The model under review builds one solid part; all positions refer to its coordinate system, in mm. Coordinates: 2 decimals unless noted, no trailing zeros. Loops run counter-clockwise (first coordinate to the right, second up) from the corner with the lowest first, then second, coordinate; pieces in that order, holes last. Notation, with made-up numbers: M 8.25,-21 L 32.25,-21 A18 cw 32.25,5 Z; hole C -6.75,-32.5 d3. An arc over 180 degrees is marked long. One line per item, written item: value.
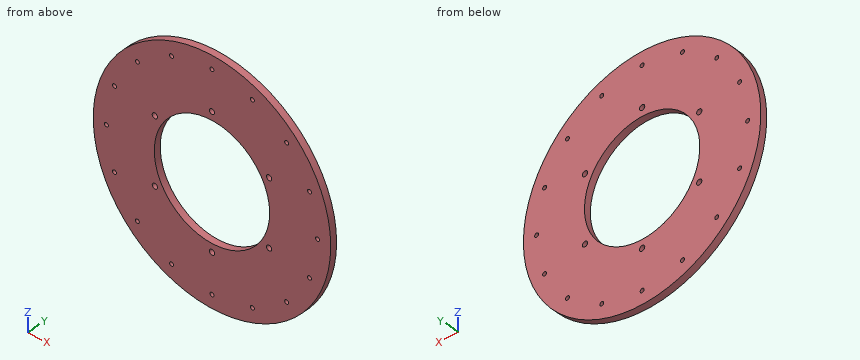
```python
from build123d import *

# Parameters (mm, degrees)
SKETCH1_R           = 180
SKETCH1_R_2         = 87.5
SKETCH1_R_3         = 3
SKETCH1_R_4         = 4
BOSS_EXTRUDE1_DEPTH = 10


with BuildPart() as part:
    # Sketch1 → Boss-Extrude1 (new body)
    with BuildSketch(Plane(origin=(0, 0, 0), x_dir=(1, 0, 0), z_dir=(0, 1, 0))):
        Circle(SKETCH1_R)
        Circle(SKETCH1_R_2, mode=Mode.SUBTRACT)
        with Locations((0, 160)):
            Circle(SKETCH1_R_3, mode=Mode.SUBTRACT)
        with Locations((61.229349178, 147.820725202)):
            Circle(SKETCH1_R_3, mode=Mode.SUBTRACT)
        with Locations((113.13708499, 113.13708499)):
            Circle(SKETCH1_R_3, mode=Mode.SUBTRACT)
        with Locations((147.820725202, 61.229349178)):
            Circle(SKETCH1_R_3, mode=Mode.SUBTRACT)
        with Locations((160, 0)):
            Circle(SKETCH1_R_3, mode=Mode.SUBTRACT)
        with Locations((147.820725202, -61.229349178)):
            Circle(SKETCH1_R_3, mode=Mode.SUBTRACT)
        with Locations((113.13708499, -113.13708499)):
            Circle(SKETCH1_R_3, mode=Mode.SUBTRACT)
        with Locations((61.229349178, -147.820725202)):
            Circle(SKETCH1_R_3, mode=Mode.SUBTRACT)
        with Locations((0, -160)):
            Circle(SKETCH1_R_3, mode=Mode.SUBTRACT)
        with Locations((-61.229349178, -147.820725202)):
            Circle(SKETCH1_R_3, mode=Mode.SUBTRACT)
        with Locations((-113.13708499, -113.13708499)):
            Circle(SKETCH1_R_3, mode=Mode.SUBTRACT)
        with Locations((-147.820725202, -61.229349178)):
            Circle(SKETCH1_R_3, mode=Mode.SUBTRACT)
        with Locations((-160, 0)):
            Circle(SKETCH1_R_3, mode=Mode.SUBTRACT)
        with Locations((-147.820725202, 61.229349178)):
            Circle(SKETCH1_R_3, mode=Mode.SUBTRACT)
        with Locations((-113.13708499, 113.13708499)):
            Circle(SKETCH1_R_3, mode=Mode.SUBTRACT)
        with Locations((-61.229349178, 147.820725202)):
            Circle(SKETCH1_R_3, mode=Mode.SUBTRACT)
        with Locations((0, 100)):
            Circle(SKETCH1_R_4, mode=Mode.SUBTRACT)
        with Locations((86.602540378, 50)):
            Circle(SKETCH1_R_4, mode=Mode.SUBTRACT)
        with Locations((86.602540378, -50)):
            Circle(SKETCH1_R_4, mode=Mode.SUBTRACT)
        with Locations((0, -100)):
            Circle(SKETCH1_R_4, mode=Mode.SUBTRACT)
        with Locations((-86.602540378, -50)):
            Circle(SKETCH1_R_4, mode=Mode.SUBTRACT)
        with Locations((-86.602540378, 50)):
            Circle(SKETCH1_R_4, mode=Mode.SUBTRACT)
    extrude(amount=BOSS_EXTRUDE1_DEPTH)


solid = part.part
```
(1) Add section C-C on z = 128. State the section outline as (x, y) points, then the cut area to 3 significant figures.
Checks:
outline: M -126.55,0 L 126.55,0 L 126.55,10 L -126.55,10 Z
area: 2,530 mm^2
(2) To check wall thickness, follow L1, parallel to Z at x = 0, y = 2.5; L2, parallel to Z at x = -114, y = 1.25; L3, parallel to X at y = 1.5, z = -50. State the ranges of each line that lie inside material, in increasing order. Write a range as [from, to].
Checks:
L1: [-180, -163], [-157, -104], [-96, -87.5], [87.5, 96], [104, 157], [163, 180]
L2: [-139.3, -116.01], [-110.26, 110.26], [116.01, 139.3]
L3: [-172.92, -90.6], [-82.6, -71.81], [71.81, 82.6], [90.6, 172.92]
(3) Add section D-D on x = 126. State the section outline as (y, z) points.
Checks:
outline: M 0,-128.55 L 10,-128.55 L 10,128.55 L 0,128.55 Z
(4) Add section A-A on x = 20. State the section outline as (y, z) points.
Checks:
outline: M 0,-178.89 L 10,-178.89 L 10,-85.18 L 0,-85.18 Z; M 0,85.18 L 10,85.18 L 10,178.89 L 0,178.89 Z
(5) Add section B-B on y = 2.5. State how many separate pieces and enclosed holes the cut face has, then the cut area to 3 significant figures.
Checks:
separate pieces: 1
enclosed holes: 23
area: 77,000 mm^2
(6) Insertion check: pin 1 Ø4 at (x, y) = (38.5, 7.5) entering from -Z; pin 2 Ø2 at (x, y) = (60, 8) entering from +Z; pin 3 Ø1 at (y, z) = (2.5, -115.5) entering from -X. Each pin has a flat end and moves straight along its axis. Give the tip position at first contact, or say it passes through.
Checks:
pin 1: z = -176.26
pin 2: z = 170.06
pin 3: x = -138.47
